Autodesk Inventor part; units mm, degrees
ref_plane "YZ Plane" through (0, 0, 0) normal (1, 0, 0) x (0, 1, 0)
ref_plane "XZ Plane" through (0, 0, 0) normal (0, 1, 0) x (-1, 0, 0)
ref_plane "XY Plane" through (0, 0, 0) normal (0, 0, 1) x (1, 0, 0)
sketch "Sketch4" plane through (0, 0, 0) normal (1, 0, 0) x (0, 1, 0)
  line L0 (0, 0) -> (31.75, 0)
  line L1 (31.75, 0) -> (31.75, -38.1)
  line L2 (31.75, -38.1) -> (0, -38.1)
  line L3 (0, -38.1) -> (0, 0)
  line L4 (25.4, -6.35) -> (6.35, -6.35)
  line L5 (6.35, -6.35) -> (6.35, -12.7)
  line L6 (6.35, -12.7) -> (25.4, -12.7)
  line L7 (25.4, -12.7) -> (25.4, -6.35)
  line L8 (25.4, -25.4) -> (6.35, -25.4)
  line L9 (6.35, -25.4) -> (6.35, -31.75)
  line L10 (6.35, -31.75) -> (25.4, -31.75)
  line L11 (25.4, -31.75) -> (25.4, -25.4)
  dimension "d36" = 31.75
  dimension "d37" = 38.1
  dimension "d38" = 19.05
  dimension "d39" = 6.35
  dimension "d40" = 6.35
  dimension "d41" = 6.35
  dimension "d42" = 6.35
  dimension "d43" = 6.35
  dimension "d44" = 6.35
extrude "Extrusion3" add sketch "Sketch4" along normal blind 6.35
sketch "Sketch5" plane through (6.35, 0, 0) normal (1, 0, 0) x (0, 0, -1)
  line L0 (25.4, 25.4) -> (31.75, 25.4)
  line L1 (31.75, 25.4) -> (31.75, 6.35)
  line L2 (31.75, 6.35) -> (25.4, 6.35)
  line L3 (25.4, 6.35) -> (25.4, 25.4)
  line L4 (6.35, 25.4) -> (12.7, 25.4)
  line L5 (12.7, 25.4) -> (12.7, 6.35)
  line L6 (12.7, 6.35) -> (6.35, 6.35)
  line L7 (6.35, 6.35) -> (6.35, 25.4)
  line L8 (0, 31.75) -> (0, 0)
  line L9 (0, 0) -> (38.1, 0)
  line L10 (38.1, 0) -> (38.1, 31.75)
  line L11 (38.1, 31.75) -> (0, 31.75)
  circle A0 centre (19.05, 15.875) radius 4.7625
  dimension "d47" = 9.525
extrude "Extrusion4" cut sketch "Sketch5" against normal blind 3.175 contours A0
sketch "Sketch6" plane through (0, 0, 0) normal (0, 0, 1) x (1, 0, 0)
  line L0 (3.175, 20.6375) -> (3.175, 11.1125)
  line L1 (0, 0) -> (0, 31.75)
  line L2 (0, 0) -> (6.35, 0)
  line L3 (6.35, 31.75) -> (6.35, 0)
  line L4 (0, 31.75) -> (6.35, 31.75)
  line L5 (0, 0) -> (6.35, 0)
  line L6 (0, 0) -> (31.75, 0)
  line L7 (31.75, 0) -> (31.75, 31.75)
  line L8 (31.75, 31.75) -> (0, 31.75)
  line L9 (0, 31.75) -> (0, 0)
  circle A0 centre (25.9588, 28.0162) radius 2.159
  circle A1 centre (25.9588, 3.7338) radius 2.159
  circle A2 centre (12.1412, 28.0162) radius 2.159
  circle A3 centre (12.1415, 3.8174) radius 2.159
  dimension "d50" = 31.75
  dimension "d51" = 4.318
  dimension "d53" = 3.7338
  dimension "d54" = 5.7912
  dimension "d55" = 4.318
  dimension "d56" = 4.318
  dimension "d57" = 4.318
  dimension "d58" = 13.8176
  dimension "d59" = 3.7338
  dimension "d60" = 13.8176
  dimension "d61" = 5.7912
  dimension "d64" = 3.7338
extrude "Extrusion5" add sketch "Sketch6" against normal blind 6.35 contours L3 L8 L7 L6
properties part number "TensionerPlate"
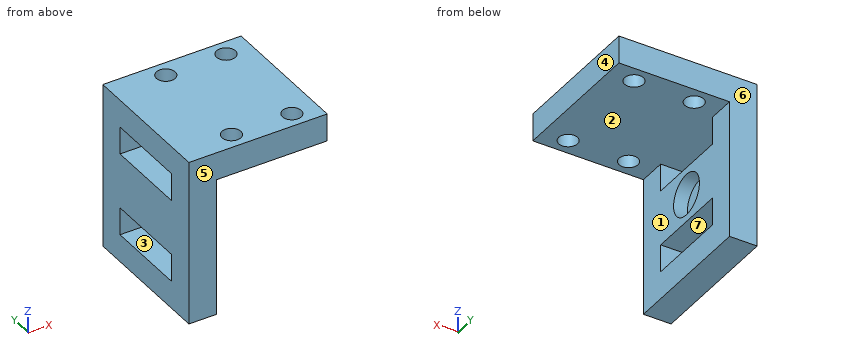
Source: CAD feature listing. Evaluate the final solid. Frame: model axes, mm. Face numbers are marked on the shaded views. A direction names the side the tool comes from. Round coordinates to 2 decimals unless told otherwise and drop trailing zeros. Order: outer loops, then holes, each group sorted by start corner. A loop starts at its lowest first (then second) coordinate and runs counter-clockwise, first axis right, second up. Notation, with made-up numbers: (6, 7.25) -> (42, 7.25) arc R14 cw to (42, 33.25) -> close; hole circle Ø9 at (3, 48.25). An arc over 180 degrees is marked (long way). Use CSV: the item, a comma, the result in double quotes.
(1) Ray query, L1, parallel to Y at x = 27, z = -6; L2, parallel to X at y = 8, z = -14; L3, parallel to Y at x = 12.5, z = -4.5. Return the intervals inside material, ascending.
Report:
L1,"0 to 1.84, 5.63 to 26.12, 29.91 to 31.75"
L2,"0 to 6.35"
L3,"0 to 1.69, 5.95 to 25.89, 30.15 to 31.75"
(2) Pull-direction query (Y, two-part tool) for the marked faces 4, 5, 6 and 7; classes: +Y half, -Y half, draft (parallel to the pull), parting line (faces both ways), or undercut.
Report:
face 4,"draft"
face 5,"-Y half"
face 6,"+Y half"
face 7,"undercut"
(3) First-contact query: pin 1 Ø10.5 at (y, z) = (14, -20) entering from +X; pin 2 Ø5 at (x, y) = (12.14, 28.02) entering from -Z; pin 3 Ø2.5 at (x, y) = (25.96, 28.02) entering from -Z. Flat tips, straight axial feed; report the tip coordinate or a pass-through.
Report:
pin 1,"x = 6.35"
pin 2,"z = -6.35"
pin 3,"through"
(4) Access query for the marked faces 1, 2 and 3. Directions: +Z, -Z, +X, -X, +Y, -Y. A direction counts if a zero-diameter tool reaches every point of the face in a straight line with its end or side. Return the directions, or none.
Report:
face 1,"-Z, +X, +Y, -Y"
face 2,"+X"
face 3,"+X, -X"
(5) Section C-C on x = 12. Return the cut outline in (y, z), and give its area (3 significant figures).
Report:
outline,"(0, -6.35) -> (1.66, -6.35) -> (1.66, 0) -> (0, 0) -> close; (5.97, -6.35) -> (25.86, -6.35) -> (25.86, 0) -> (5.97, 0) -> close; (30.17, -6.35) -> (31.75, -6.35) -> (31.75, 0) -> (30.17, 0) -> close"
area,"147 mm^2"
(6) Section B-B on y = 22.5. Return the cut outline in (x, z).
Report:
outline,"(0, -38.1) -> (6.35, -38.1) -> (6.35, -31.75) -> (0, -31.75) -> close; (0, -25.4) -> (6.35, -25.4) -> (6.35, -12.7) -> (0, -12.7) -> close; (0, -6.35) -> (31.75, -6.35) -> (31.75, 0) -> (0, 0) -> close"
(7) Section A-A on z = -31. Return the cut outline in (x, y).
Report:
outline,"(0, 0) -> (6.35, 0) -> (6.35, 6.35) -> (0, 6.35) -> close; (0, 25.4) -> (6.35, 25.4) -> (6.35, 31.75) -> (0, 31.75) -> close"
